Can you work these out from the model? Positions are in its coordinate system, mm. A direction names the side the tool comes from. Give positions to 0.01 mm unless a question says otherwise; leave off trailing zeros. Loops run counter-clockwise (first coordinate to the right, second up) from the corner with the lowest first, then second, coordinate; pieces in that order, holes last. Notation, with made-up numbers: M 82.5,83.25 L 106.5,83.25 A24 ccw 106.5,98.25 Z; hole C -4.75,53.5 d9. An arc over 180 degrees is marked long. Put each result on its own line as item: value. Start each with the question number.
1) Imagine slicing it at A-A (z = 3.75). Write out the boundary of the cut face in (x, y), then the cut area to 3 significant figures.
2) If we mould it in two halves opening along X, with no side actions, what happens to faces 4 (the flat face through (-34.98, 26.01, 7.51)), 5 (the flat face through (-44, 36, 0)), 6 (the cylindrical face through (-49.66, 40.64, 10.09))? For each: +X half, -X half, draft (parallel to the pull), parting line (faces both ways), or undercut.
3) Imagine slicing it at B-B (z = 13.75). Write out the boundary of the cut face in (x, y) (1 decimal), then the cut area to 3 significant figures.
4) For faces 1 (the flat face through (-36.2, 24.8, 15.24)), 2 (the flat face through (-41.36, 24.9, 7.51)), 3 (the flat face through (-35, 17, 5.08)), which set-ups out of +Z, -Z, +X, -X, +Y, -Y let a thin tool reach every point of the face, with its end or its side?
5) For P1, Ø2, axis at y = 36.5, z = 8.5, coming from the -X side; P2, Ø1, axis at x = -34, z = 9.5, coming from the -Y side; P3, Ø8, axis at y = 27.5, z = 11, coming from the +X side, each with a flat end and sliding along its axis, tell me the tip position at first contact or that it passes through.
6) Please list where these lines run through material, in increasing order: line 1 along Z through (x, y) = (-52.5, 23); line 2 along X through (y, z) = (31, 1.75); line 3 along X through (y, z) = (32, 8.25). Write a range as from..to.
from build123d import *

# Parameters (mm, degrees)
F0_R     = 21.59
F0_R_2   = 14.2875
F1_DEPTH = 5.08
F1_TAPER = -3
F2_DEPTH = 15.24


with BuildPart() as f1:
    # F0 (on Top) → F1 (new body)
    with BuildSketch(Plane.XY):
        with Locations((-39.1328502254, 30.9806439229)):
            Circle(F0_R)
        with Locations((-39.1328502254, 30.9806439229)):
            Circle(F0_R_2, mode=Mode.SUBTRACT)
    extrude(amount=F1_DEPTH, taper=F1_TAPER)

    # F0 (on Top) → F2 (join)
    with BuildSketch(Plane.XY):
        with Locations((-39.1328502254, 30.9806439229)):
            Circle(F0_R_2)
        Polygon((-40.3579410266, 38.3586195618), (-33.3558812942, 35.7305914981), (-32.130790493, 28.3526158592), (-37.9077594242, 23.602668284), (-44.9098191566, 26.2306963477), (-46.1349099578, 33.6086719866), align=None, mode=Mode.SUBTRACT)
    extrude(amount=F2_DEPTH)


solid = f1.part
Recorded:
1. outline: C -39.13,30.98 d43.57; hole M -46.13,33.61 L -44.91,26.23 L -37.91,23.6 L -32.13,28.35 L -33.36,35.73 L -40.36,38.36 Z
1. area: 1,350 mm²
2. face 4: undercut
2. face 5: draft
2. face 6: parting line
3. outline: C -39.1,31 d28.6; hole M -46.1,33.6 L -44.9,26.2 L -37.9,23.6 L -32.1,28.4 L -33.4,35.7 L -40.4,38.4 Z
3. area: 496 mm²
4. face 1: +Z, +X, -X, +Y, -Y
4. face 2: +Z, -Z
4. face 3: +Z
5. P1: x = -52.69
5. P2: y = 17.47
5. P3: x = -24.85
6. line 1: 0..5.08
6. line 2: -60.81..-45.7, -32.57..-17.45
6. line 3: -53.38..-45.87, -32.74..-24.88
